For this review, use the dimensioned drawing (mm, ordinates from the lowest corner) and the shaded views. Give positions to 0.01 mm unless a question says otherwise; leave off trailing zeros. Order: outer loops, then holes, each group sorted by start corner. A loop starts at its lowest first (then second) coordinate and runs counter-clockwise, first axis right, second up. Notation, with made-up numbers: (86, -34) - (91, -34) arc R17 cw to (91, -30) - close; hole circle Ø7 at (60.5, 15.5). An arc over 180 degrees is marked (long way). Use a Markdown table: item, result. Add a question column.
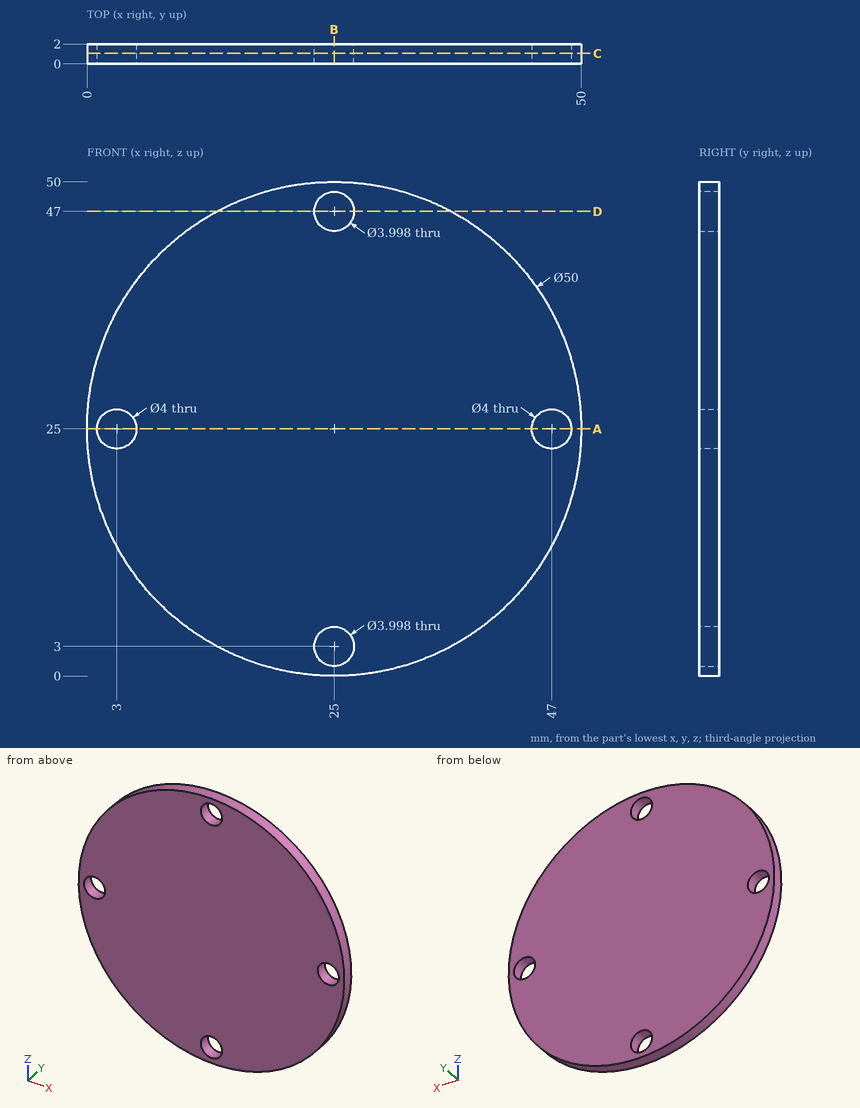
Q1. Wall thickness on probe 1 along X at (y, z) = (0.6, 25); probe 2 along Z at (x, y) = (25.5, 1.6) (1 decimal); probe 3 along X at (y, z) = (1.15, 47) (1 decimal): over which ranges is each line inside the solid? List them lowest first.
Q2. We need section B-B (x = 25). Write out the cut boundary in (y, z).
Q3. We need section C-C (y = 1.05). Write out the cut boundary in (x, z), plus the area to 3 significant figures.
Q4. We need section A-A (z = 25). Write out the cut boundary in (x, y).
Q5. We need section D-D (z = 47). Write out the cut boundary in (x, y) (1 decimal).
Here are the results:
| question | item | result |
|---|---|---|
| 1 | probe 1 | 0 to 1, 5 to 45, 49 to 50 |
| 1 | probe 2 | 0 to 1.1, 4.9 to 45.1, 48.9 to 50 |
| 1 | probe 3 | 13.1 to 23, 27 to 36.9 |
| 2 | outline | (0, 0) - (2, 0) - (2, 1) - (0, 1) - close; (0, 5) - (2, 5) - (2, 45) - (0, 45) - close; (0, 49) - (2, 49) - (2, 50) - (0, 50) - close |
| 3 | outline | circle Ø50 at (25, 25); hole circle Ø4 at (3, 25); hole circle Ø4 at (25, 3); hole circle Ø4 at (25, 47); hole circle Ø4 at (47, 25) |
| 3 | area | 1,910 mm2 |
| 4 | outline | (0, 0) - (1, 0) - (1, 2) - (0, 2) - close; (5, 0) - (45, 0) - (45, 2) - (5, 2) - close; (49, 0) - (50, 0) - (50, 2) - (49, 2) - close |
| 5 | outline | (13.1, 0) - (23, 0) - (23, 2) - (13.1, 2) - close; (27, 0) - (36.9, 0) - (36.9, 2) - (27, 2) - close |
